Here's how the part is built. I have some questions about the finished solid (model axes, mm). Give positions to 0.01 mm unless a question says otherwise; leave off trailing zeros. Write each loop counter-clockwise with the first axis right and the second up, starting at its lowest first coordinate (ties: lowest second). Pieces come first, ordered by that corner, then holes. Notation, with made-up numbers: (-14, 30.5) - (3, 30.5) arc R35 cw to (3, 69.5) - close; hole circle Ø7 at (-38, -32). An arc over 180 degrees is marked (long way). Use a Markdown table: item, result.
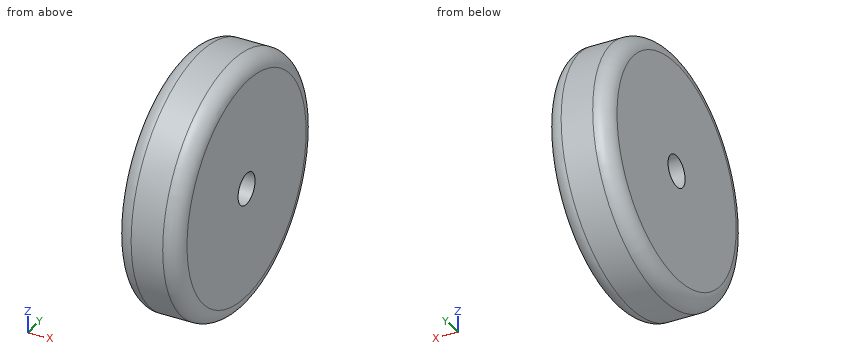
```python
from build123d import *

# Parameters (mm, degrees)
F0_R     = 101.6
F1_DEPTH = 25.4
F2_R     = 12.7
F3_R     = 12.7
F4_DEPTH = 50.801


with BuildPart() as f1:
    # F0 (on Right) → F1 (new body, symmetric)
    with BuildSketch(Plane.YZ):
        Circle(F0_R)
    extrude(amount=F1_DEPTH, both=True)

    # F2
    f2_edges = [f1.edges().sort_by_distance(p)[0] for p in [
        (-25.4, -101.6, 0),
        (25.4, -101.6, 0),
    ]]
    fillet(f2_edges, radius=F2_R)

    # F3 (on face) → F4 (cut, through all)
    with BuildSketch(Plane(origin=(-25.4, 0, 0), x_dir=(0, -1, 0), z_dir=(-1, 0, 0))):
        Circle(F3_R)
    extrude(amount=-F4_DEPTH, mode=Mode.SUBTRACT)


solid = f1.part
```
Item 1: Will these pins go through, and if not, where does the flat tip stop? pin 1 Ø1.5 at (x, z) = (-4, 16) entering from +Y; pin 2 Ø1 at (x, z) = (-5.5, -48) entering from -Y; pin 3 Ø12 at (x, z) = (18.5, 54) entering from +Y.
Values:
| item | result |
|---|---|
| pin 1 | stops at y = 100.45 |
| pin 2 | stops at y = -89.81 |
| pin 3 | stops at y = 88.76 |
Item 2: If we section it at C-C, the plane x = -3.5: Write out the boundary of the cut face in (y, z), plus the area to 3 significant figures.
Values:
| item | result |
|---|---|
| outline | circle Ø203.2 at (0, 0); hole circle Ø25.4 at (0, 0) |
| area | 31,900 mm2 |
Item 3: If we section it at D-D, the plane x = 22: Write out the boundary of the cut face in (y, z).
Values:
| item | result |
|---|---|
| outline | circle Ø195.1 at (0, 0); hole circle Ø25.4 at (0, 0) |
Item 4: If we section it at A-A, the plane z = 0: Write out the boundary of the cut face in (x, y).
Values:
| item | result |
|---|---|
| outline | (-25.4, -88.9) arc R12.7 ccw to (-12.7, -101.6) - (12.7, -101.6) arc R12.7 ccw to (25.4, -88.9) - (25.4, -12.7) - (-25.4, -12.7) - close; (-25.4, 12.7) - (25.4, 12.7) - (25.4, 88.9) arc R12.7 ccw to (12.7, 101.6) - (-12.7, 101.6) arc R12.7 ccw to (-25.4, 88.9) - close |
Item 5: I need wall thicknesses on line 1 along Z through (x, y) = (10, 0); line 2 along X through (y, z) = (-86.5, 22); line 3 along X through (y, z) = (-55.5, -81.5). Which ranges of each line are inside material? Lowest first, please. Write a range as [from, to].
Values:
| item | result |
|---|---|
| line 1 | z = [-101.6, -12.7], [12.7, 101.6] |
| line 2 | x = [-25.4, 25.4] |
| line 3 | x = [-20.89, 20.89] |
